Geometry: see drawing. Coordinates: mm, zero at the bounding-box minimum. A direction names the side the tool comes from. Give positions to 0.01 mm unless a question says otherwise; leave off trailing zeros. Loops run counter-clockwise (first coordinate to the right, second up) from the corner with the lowest first, then second, coordinate; pieces in that order, holes last. Notation, with made-up numbers: M 5,84 L 54,84 A12 cw 54,100 Z; hole C -25,36 d2. An arc over 180 degrees is marked long. Answer in a Markdown table with one row per item.
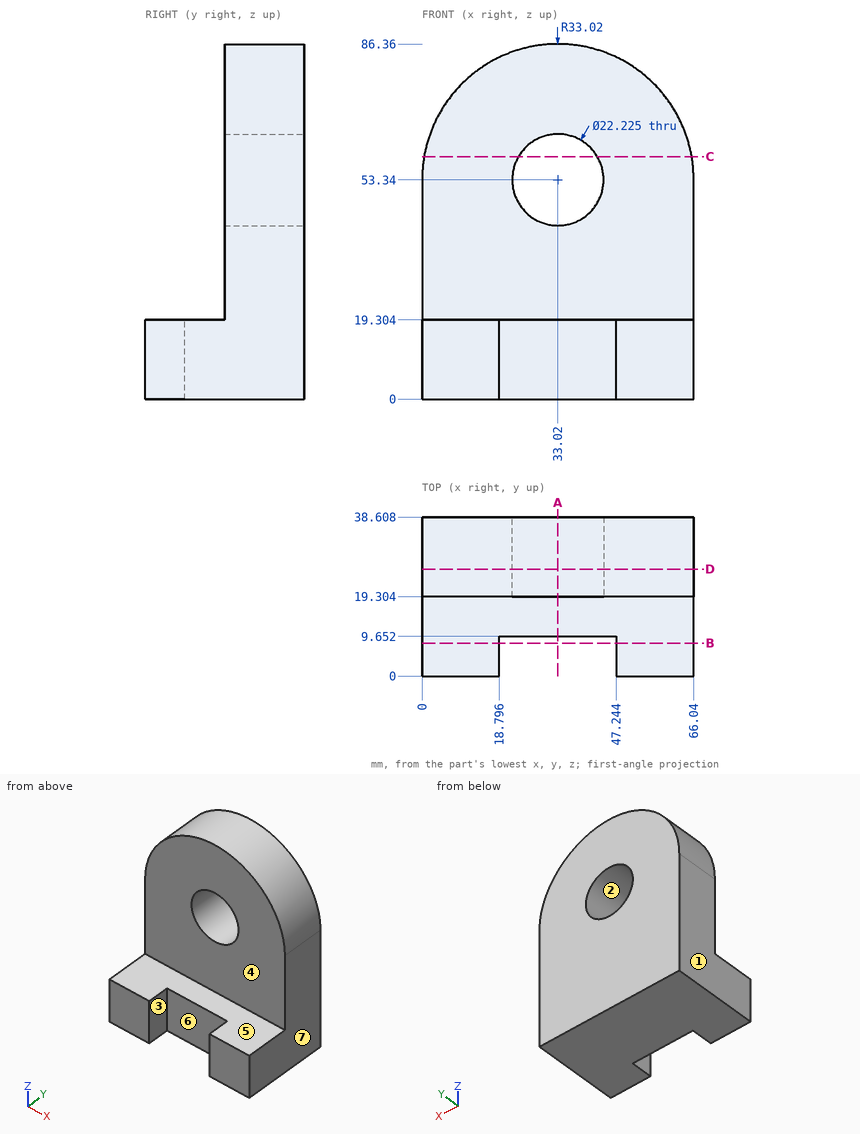
1) Section D-D, the plane y = 26. Return loops of the section in (x, z) (1 decimal), then the cut area to 3 significant figures.
Reply:
| item | result |
|---|---|
| outline | M 0,0 L 66,0 L 66,53.3 A33 ccw 0,53.3 Z; hole C 33,53.3 d22.2 |
| area | 4,850 mm² |
2) Section B-B, the plane y = 8. Return loops of the section in (x, z).
Reply:
| item | result |
|---|---|
| outline | M 0,0 L 18.8,0 L 18.8,19.3 L 0,19.3 Z; M 47.24,0 L 66.04,0 L 66.04,19.3 L 47.24,19.3 Z |
3) Pull-direction query (X, two-part tool) for the marked faces 1, 2, 3 and 4; classes: released by +X, released by -X, zero draft, split by the parting line, or undercut.
Reply:
| item | result |
|---|---|
| face 1 | released by -X |
| face 2 | undercut |
| face 3 | undercut |
| face 4 | zero draft |
4) Material intervals for L1, parallel to Z at x = 33, y = 25; L2, parallel to X at y = 26, z = 53; L3, parallel to Y at x = 53.5, z = 71, sorted ascending.
Reply:
| item | result |
|---|---|
| L1 | z = 0 to 42.23, 64.45 to 86.36 |
| L2 | x = 0 to 21.91, 44.13 to 66.04 |
| L3 | y = 19.3 to 38.61 |
5) Set-up query: the marked faces 5, 6 and 7. Return all of +Z, -Z, +X, -X, +Y, -Y with unobstructed straight access to the full face (end or side cutting, diameter ignored); none if empty.
Reply:
| item | result |
|---|---|
| face 5 | +Z, +X, -X, -Y |
| face 6 | +Z, -Z, -Y |
| face 7 | +Z, -Z, +X, +Y, -Y |
6) Section A-A, the plane x = 33.02. Return loops of the section in (y, z).
Reply:
| item | result |
|---|---|
| outline | M 9.65,0 L 38.61,0 L 38.61,42.23 L 19.3,42.23 L 19.3,19.3 L 9.65,19.3 Z; M 19.3,64.45 L 38.61,64.45 L 38.61,86.36 L 19.3,86.36 Z |
7) Pin query (flat end, axial travel): pin 1 Ø6 at (x, z) = (29.5, 6) entering from -Y; pin 2 Ø8 at (x, z) = (45.5, 19.5) entering from -Y; pin 3 Ø12 at (x, z) = (31.5, 53.5) entering from +Y; pin 4 Ø9.5 at (x, y) = (18, 12) entering from +Z. Return the tip coordinate at first contact, or that it passes through.
Reply:
| item | result |
|---|---|
| pin 1 | stops at y = 9.65 |
| pin 2 | stops at y = 0 |
| pin 3 | passes through |
| pin 4 | stops at z = 19.3 |
8) Section C-C, the plane z = 59. Return loops of the section in (x, y).
Reply:
| item | result |
|---|---|
| outline | M 0.49,19.3 L 23.46,19.3 L 23.46,38.61 L 0.49,38.61 Z; M 42.58,19.3 L 65.55,19.3 L 65.55,38.61 L 42.58,38.61 Z |
